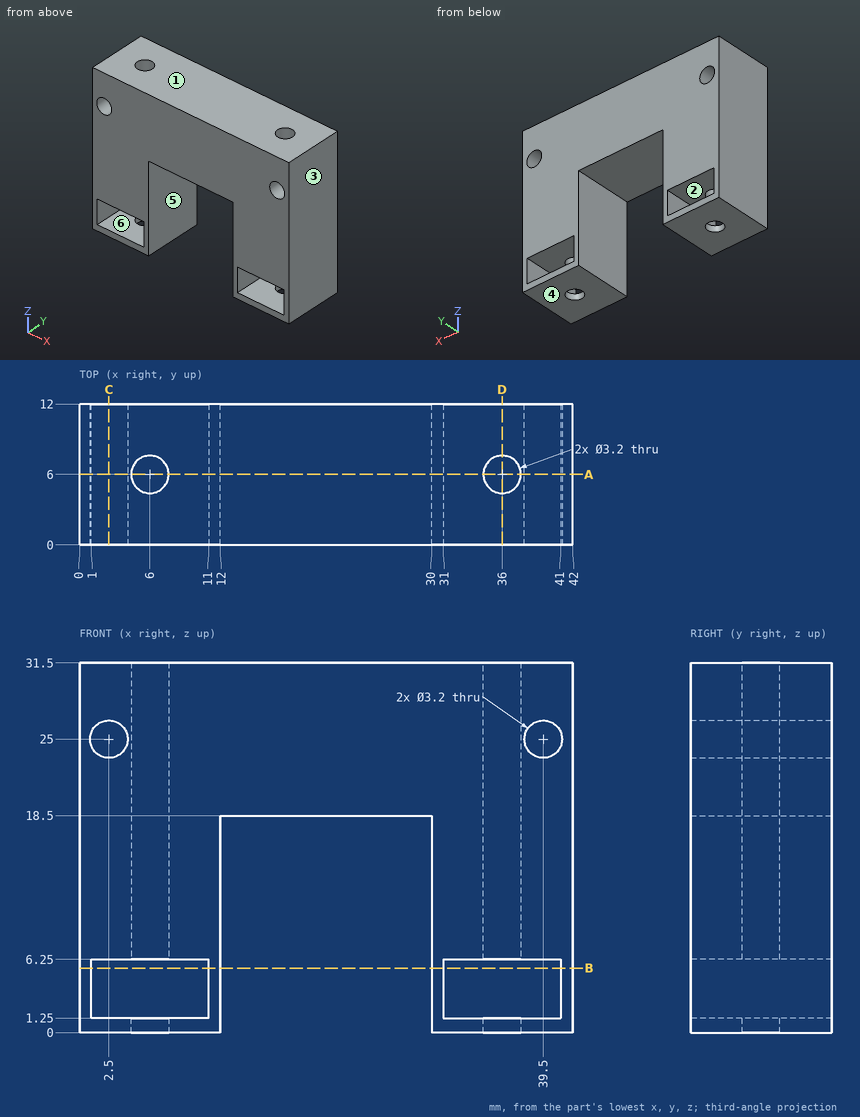
Design review of the part shown in the three views and the two pictorial views. Dimensions are in mm from the part's minimum x, y and z. A direction names the side the tool comes from. Round coordinates to 2 decimals unless told otherwise and drop trailing zeros. Write each loop counter-clockwise with the first axis right and the second up, starting at its lowest first coordinate (ties: lowest second). Pieces come first, ordered by that corner, then holes.
1) Take a section at C-C on x = 2.5. Give the boundary of the cut face in (y, z), then the cut area to 3 significant figures.
Answer below:
outline: (0, 0) - (12, 0) - (12, 1.25) - (0, 1.25) - close; (0, 6.25) - (12, 6.25) - (12, 23.4) - (0, 23.4) - close; (0, 26.6) - (12, 26.6) - (12, 31.5) - (0, 31.5) - close
area: 280 mm2
2) For line 1 along X through (y, z) = (2.5, 2); line 2 along Z through (x, y) = (39.5, 7.75); line 3 along X through (y, z) = (3, 25), list the stretches that pass through material, from the lowest coordinate up.
Answer below:
line 1: x = 0 to 1, 11 to 12, 30 to 31, 41 to 42
line 2: z = 0 to 1.25, 6.25 to 23.4, 26.6 to 31.5
line 3: x = 0 to 0.9, 4.1 to 37.9, 41.1 to 42
3) Insertion check: pin 1 Ø3.5 at (x, y) = (20, 7.5) entering from -Z. The pin has a flat end and moves straight along its axis. Give the tip position at first contact, or say it passes through.
Answer below:
pin 1: stops at z = 18.5
4) Take a section at D-D on x = 36. Give the boundary of the cut face in (y, z).
Answer below:
outline: (0, 0) - (4.4, 0) - (4.4, 1.25) - (0, 1.25) - close; (0, 6.25) - (4.4, 6.25) - (4.4, 31.5) - (0, 31.5) - close; (7.6, 0) - (12, 0) - (12, 1.25) - (7.6, 1.25) - close; (7.6, 6.25) - (12, 6.25) - (12, 31.5) - (7.6, 31.5) - close
5) Take a section at B-B on z = 5.5. Give the boundary of the cut face in (x, y).
Answer below:
outline: (0, 0) - (1, 0) - (1, 12) - (0, 12) - close; (11, 0) - (12, 0) - (12, 12) - (11, 12) - close; (30, 0) - (31, 0) - (31, 12) - (30, 12) - close; (41, 0) - (42, 0) - (42, 12) - (41, 12) - close
6) Mouldability with a two-part tool opening along X and no side actions: class the marked faces 1, 2 and 3 as +X half, -X half, draft (parallel to the pull), parting line (faces both ways), or undercut.
Answer below:
face 1: draft
face 2: undercut
face 3: +X half
7) Machinability: for the marked faces 4, 5 and 6, which of the approach directions +Z, -Z, +X, -X, +Y, -Y give a long, thin tool a straight path to every point of the face, cutting with its end or side? Answer none if there is none.
Answer below:
face 4: -Z, +X, -X, +Y, -Y
face 5: -Z, +Y, -Y
face 6: +Y, -Y
8) Take a section at A-A on y = 6. State how many separate pieces and enclosed holes the cut face has, then the cut area to 3 significant figures.
Answer below:
separate pieces: 3
enclosed holes: 2
area: 704 mm2
